from build123d import *

# Parameters (mm, degrees)
CROQUIS1_W              = 200
CROQUIS1_H              = 170
SALIENTE_EXTRUIR1_DEPTH = 10
CROQUIS2_W              = 59.79
CROQUIS2_H              = 10
CROQUIS2_W_2            = 30.21
SALIENTE_EXTRUIR2_DEPTH = 150
CROQUIS3_W              = 90
CROQUIS3_H              = 10
SALIENTE_EXTRUIR3_DEPTH = 100
CROQUIS4_W              = 5.25
CROQUIS4_H              = 5.5
CORTAR_EXTRUIR1_DEPTH   = 170
CROQUIS7_W              = 90
CROQUIS7_H              = 10
SALIENTE_EXTRUIR4_DEPTH = 5
CORTAR_EXTRUIR3_DEPTH   = 10
CORTAR_EXTRUIR4_DEPTH   = 30
CORTAR_EXTRUIR5_DEPTH   = 5
CROQUIS10_W             = 30
CROQUIS10_H             = 13.5
CROQUIS10_W_2           = 24
CROQUIS10_H_2           = 8
SALIENTE_EXTRUIR5_DEPTH = 4.3
CROQUIS11_R             = 1.1
CORTAR_EXTRUIR6_DEPTH   = 14.3
CROQUIS12_R             = 1.75
CORTAR_EXTRUIR7_DEPTH   = 6.4
CROQUIS13_R             = 1.7
CORTAR_EXTRUIR8_DEPTH   = 5
CROQUIS14_W             = 0.3
CROQUIS14_H             = 10
CORTAR_EXTRUIR9_DEPTH   = 5
SALIENTE_EXTRUIR6_DEPTH = 5
CROQUIS16_W             = 200
CROQUIS16_H             = 160
CORTAR_EXTRUIR10_DEPTH  = 162
CROQUIS16_2_W           = 200
CROQUIS16_2_H           = 160
CORTAR_EXTRUIR11_DEPTH  = 162


with BuildPart() as part:
    # Croquis1 → Saliente-Extruir1 (new body)
    with BuildSketch(Plane(origin=(0, 0, 0), x_dir=(1, 0, 0), z_dir=(0, 1, 0))):
        Rectangle(CROQUIS1_W, CROQUIS1_H)
    extrude(amount=SALIENTE_EXTRUIR1_DEPTH)

    # Croquis2 → Saliente-Extruir2 (add)
    with BuildSketch(Plane(origin=(0, 10, 0), x_dir=(1, 0, 0), z_dir=(0, 1, 0))):
        Polygon((-100, 85), (-100, -85), (-90, -85), (-90, -75), (-90, 75), (-90, 85), align=None)
        Polygon((100, 85), (90, 85), (90, 75), (90, -75), (90, -85), (100, -85), align=None)
        with Locations((-60.105, -80)):
            Rectangle(CROQUIS2_W, CROQUIS2_H)
        with Locations((74.895, -80)):
            Rectangle(CROQUIS2_W_2, CROQUIS2_H)
    extrude(amount=SALIENTE_EXTRUIR2_DEPTH)

    # Croquis3 → Saliente-Extruir3 (add)
    with BuildSketch(Plane(origin=(0, 160, 0), x_dir=(1, 0, 0), z_dir=(0, 1, 0))):
        with Locations((14.79, -80)):
            Rectangle(CROQUIS3_W, CROQUIS3_H)
    extrude(amount=-SALIENTE_EXTRUIR3_DEPTH)

    # Croquis4 → Cortar-Extruir1 (cut)
    with BuildSketch(Plane(origin=(0, 10, 65), x_dir=(-1, 0, 0), z_dir=(0, 1, 0))):
        with Locations((92.625, -145)):
            Rectangle(CROQUIS4_W, CROQUIS4_H)
        with Locations((-92.625, -145)):
            Rectangle(CROQUIS4_W, CROQUIS4_H)
    extrude(amount=CORTAR_EXTRUIR1_DEPTH, mode=Mode.SUBTRACT)

    # Croquis7 → Saliente-Extruir4 (add)
    with BuildSketch(Plane.XY.offset(85)):
        with Locations((14.79, 65)):
            Rectangle(CROQUIS7_W, CROQUIS7_H)
    extrude(amount=SALIENTE_EXTRUIR4_DEPTH)

    # Croquis8 → Cortar-Extruir3 (cut)
    with BuildSketch(Plane(origin=(0, 160, 0), x_dir=(1, 0, 0), z_dir=(0, 1, 0))):
        Polygon((98, 70), (98, -83), (-98, -83), (-98, 70), (-92, 70), (-92, -77), (92, -77), (92, 70), align=None)
    extrude(amount=-CORTAR_EXTRUIR3_DEPTH, mode=Mode.SUBTRACT)

    # Croquis9 → Cortar-Extruir4 (cut)
    with BuildSketch(Plane(origin=(0, 10, 0), x_dir=(1, 0, 0), z_dir=(0, 1, 0))):
        Polygon((-95.25, 77.25), (-95.25, 82.75), (-71.25, 82.75), (-71.25, 77.25), (-71.25, 74.75), (-95.25, 74.75), align=None)
    extrude(amount=-CORTAR_EXTRUIR4_DEPTH, mode=Mode.SUBTRACT)

    # Croquis9_2 → Cortar-Extruir5 (cut)
    with BuildSketch(Plane(origin=(0, 10, 0), x_dir=(1, 0, 0), z_dir=(0, 1, 0))):
        Polygon((-95.25, 77.25), (-95.25, 82.75), (-71.25, 82.75), (-71.25, 77.25), (-71.25, 74.75), (-95.25, 74.75), align=None)
    extrude(amount=CORTAR_EXTRUIR5_DEPTH, mode=Mode.SUBTRACT)

    # Croquis10 → Saliente-Extruir5 (add)
    with BuildSketch(Plane.XZ):
        with Locations((-83.25, -78.5)):
            Rectangle(CROQUIS10_W, CROQUIS10_H)
        with Locations((-83.25, -78.75)):
            Rectangle(CROQUIS10_W_2, CROQUIS10_H_2, mode=Mode.SUBTRACT)
    extrude(amount=SALIENTE_EXTRUIR5_DEPTH)

    # Croquis11 → Cortar-Extruir6 (cut)
    with BuildSketch(Plane.XY.offset(-71.75)):
        with Locations((-77.55, -2.1)):
            Circle(CROQUIS11_R)
        with Locations((-86.93, -2.1)):
            Circle(CROQUIS11_R)
    extrude(amount=-CORTAR_EXTRUIR6_DEPTH, mode=Mode.SUBTRACT)

    # Croquis12 → Cortar-Extruir7 (cut)
    with BuildSketch(Plane.XZ):
        with Locations((-91.5, -55)):
            Circle(CROQUIS12_R)
        with Locations((18.5, -55)):
            Circle(CROQUIS12_R)
        with Locations((-91.5, 55)):
            Circle(CROQUIS12_R)
        with Locations((18.5, 55)):
            Circle(CROQUIS12_R)
    extrude(amount=-CORTAR_EXTRUIR7_DEPTH, mode=Mode.SUBTRACT)

    # Croquis13 → Cortar-Extruir8 (cut)
    with BuildSketch(Plane.XY.offset(85)):
        with Locations((-50.21, 24)):
            Circle(CROQUIS13_R)
        with Locations((79.79, 24)):
            Circle(CROQUIS13_R)
    extrude(amount=-CORTAR_EXTRUIR8_DEPTH, mode=Mode.SUBTRACT)

    # Croquis14 → Cortar-Extruir9 (cut)
    with BuildSketch(Plane.XY.offset(90)):
        with Locations((-30.06, 65)):
            Rectangle(CROQUIS14_W, CROQUIS14_H)
        with Locations((59.64, 65)):
            Rectangle(CROQUIS14_W, CROQUIS14_H)
    extrude(amount=-CORTAR_EXTRUIR9_DEPTH, mode=Mode.SUBTRACT)

    # Croquis15 → Saliente-Extruir6 (add)
    with BuildSketch(Plane.XY.offset(85)):
        Polygon((14.79, 0), (94.79, 0), (94.79, 4.8), (14.79, 4.8), (-65.21, 4.8), (-65.21, 0), align=None)
    extrude(amount=SALIENTE_EXTRUIR6_DEPTH)

    # Croquis16 → Cortar-Extruir10 (cut)
    with BuildSketch(Plane.XY.offset(85)):
        with Locations((0, 80)):
            Rectangle(CROQUIS16_W, CROQUIS16_H)
    extrude(amount=-CORTAR_EXTRUIR10_DEPTH, mode=Mode.SUBTRACT)

    # Croquis16_2 → Cortar-Extruir11 (cut)
    with BuildSketch(Plane.XY.offset(85)):
        with Locations((0, 80)):
            Rectangle(CROQUIS16_2_W, CROQUIS16_2_H)
    extrude(amount=CORTAR_EXTRUIR11_DEPTH, mode=Mode.SUBTRACT)


solid = part.part
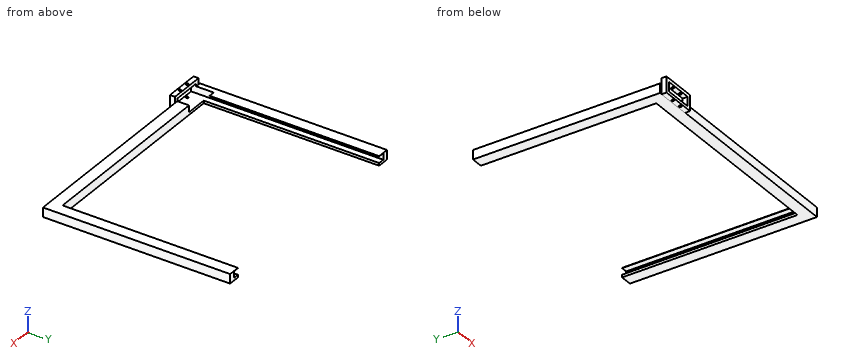
The listing builds one solid part. Answer for the finished solid, in the listing's coordinates (mm). Coordinates: 2 decimals unless noted, no trailing zeros. Write each loop counter-clockwise with the first axis right and the second up, starting at its lowest first coordinate (ties: lowest second). Pieces come first, ordered by that corner, then holes. Notation, with made-up numbers: M 89,-1.75 L 114,-1.75 A28 ccw 114,21.25 Z; hole C 44.25,-16.75 d9. An arc over 180 degrees is marked long. Use one line per item in the form item = value.
Item 1: Given P1, Ø5, axis at x = -96.5, y = 60.5, coming from the +Z side; P2, Ø2, axis at x = -86.93, y = -2.1, coming from the -Z side; P3, Ø4, axis at x = -83.5, z = -74.5, coming from the +Y side; P4, Ø1.3, axis at y = -1.5, z = -81.5, coming from the +X side, each flat-ended and moving along its own axis, determine where each tip first touches the part or whether it passes through.
Model answer:
P1 = -77
P2 = through
P3 = 0
P4 = -68.25
Item 2: Find section B-B, the plane x = -46. Give the vertices of the cut face in (y, z), plus the area to 3 significant figures.
Model answer:
outline = M 0,-85 L 10,-85 L 10,-77 L 0,-77 Z
area = 80.0 mm2
Item 3: Find the intervals of material crossed by probe 1 along X at (y, z) = (111, -78.5); probe 2 along Y at (x, z) = (-86.93, -73.65); probe 3 along Y at (x, z) = (-77.55, -84.4), in increasing order.
Model answer:
probe_1 = -100 to -95.25, 95.25 to 100
probe_2 = -4.3 to -3.2, -1 to 0
probe_3 = -4.3 to -3.2, -1 to 10
Item 4: Find section A-A, the plane y = 79. Give the vertices of the cut face in (x, z), plus the area to 3 significant figures.
Model answer:
outline = M -100,-85 L -90,-85 L -90,-82.75 L -95.25,-82.75 L -95.25,-77.25 L -90,-77.25 L -90,-77 L -100,-77 Z; M 90,-85 L 100,-85 L 100,-77 L 90,-77 L 90,-77.25 L 95.25,-77.25 L 95.25,-82.75 L 90,-82.75 Z
area = 102 mm2
